The model under review builds one solid part; all positions refer to its coordinate system, in mm. A direction names the side the tool comes from. Coordinates: 2 decimals unless noted, no trailing zeros. Loops run counter-clockwise (first coordinate to the right, second up) from the corner with the lowest first, then second, coordinate; pieces in that order, holes last. Notation, with made-up numbers: M 63,1.5 L 67,1.5 A13 ccw 67,16.5 Z; hole C 77,69.5 d11. An arc over 180 degrees is marked long. Use one line per item in the form item = value.
```python
from build123d import *

# Parameters (mm, degrees)
BOSS_EXTRUDE5_DEPTH = 3
BOSS_EXTRUDE6_START = -6
BOSS_EXTRUDE6_DEPTH = 6
CIRPATTERN4_COUNT   = 12
BOSS_EXTRUDE8_START = -9
BOSS_EXTRUDE8_DEPTH = 9
SKETCH25_R          = 27.5
SKETCH25_W          = 9
SKETCH25_H          = 25
BOSS_EXTRUDE9_DEPTH = 3
CIRPATTERN5_COUNT   = 12
FILLET2_R           = 3


with BuildPart() as part:
    # Sketch1 → Boss-Extrude5 (new body)
    with BuildSketch(Plane.XY):
        with BuildLine():
            ThreePointArc((14.753571677, -27.264117862), (12.634850146, -34.380016896), (19.750749181, -36.498738428))
            ThreePointArc((19.750749181, -36.498738428), (41.5, 0), (19.750749181, 36.498738428))
            ThreePointArc((19.750749181, 36.498738428), (12.634850146, 34.380016896), (14.753571677, 27.264117862))
            ThreePointArc((14.753571677, 27.264117862), (31, 0), (14.753571677, -27.264117862))
        make_face()
    extrude(amount=BOSS_EXTRUDE5_DEPTH)

    # Sketch1<7> → Boss-Extrude6 (add)
    with BuildSketch(Plane.XY.offset(BOSS_EXTRUDE6_START)):
        with BuildLine():
            ThreePointArc((40, 0), (33.333983987, -22.109851007), (15.557724422, -36.850470972))
            ThreePointArc((15.557724422, -36.850470972), (17.691016162, -37.113053671), (19.750749181, -36.498738428))
            ThreePointArc((19.750749181, -36.498738428), (35.650428406, -21.243750952), (41.5, 0))
            ThreePointArc((41.5, 0), (35.650428406, 21.243750952), (19.750749181, 36.498738428))
            ThreePointArc((19.750749181, 36.498738428), (17.691016162, 37.113053671), (15.557724422, 36.850470972))
            ThreePointArc((15.557724422, 36.850470972), (33.333983987, 22.109851007), (40, 0))
        make_face()
    extrude(amount=BOSS_EXTRUDE6_DEPTH)

    # Sketch23 → M4x0.7 Tapped Hole4 (revolve, cut)
    with BuildSketch(Plane(origin=(36.25, 0, 3), x_dir=(0, -1, 0), z_dir=(1, 0, 0))):
        Polygon((0, 0), (0, 11.091420021), (1.65, 10.1), (1.65, 0.375), (2.025, 0), align=None)
    m4x0_7_tapped_hole4 = revolve(axis=Axis((36.25, 0, 9.35), (0, 0, -1)), mode=Mode.SUBTRACT)

    # CirPattern4: M4x0.7 Tapped Hole4 ×12 about axis, 7 skipped
    cirpattern4_axis = Axis((0, 0, 0), (0, 0, -1))
    add([m4x0_7_tapped_hole4.rotate(cirpattern4_axis, i * 360 / CIRPATTERN4_COUNT) for i in range(1, CIRPATTERN4_COUNT) if i not in (3, 4, 5, 6, 7, 8, 9)], mode=Mode.SUBTRACT)

    # Sketch15 → Boss-Extrude8 (add)
    with BuildSketch(Plane.XY.offset(3).offset(BOSS_EXTRUDE8_START)):
        with BuildLine():
            Line((47.5, 12.5), (47.5, -12.5))
            ThreePointArc((47.5, -12.5), (39.682119593, -17.947088957), (33.186389126, -24.918137506))
            ThreePointArc((33.186389126, -24.918137506), (41.5, 0), (33.186389126, 24.918137506))
            ThreePointArc((33.186389126, 24.918137506), (39.682119593, 17.947088957), (47.5, 12.5))
        make_face()
    extrude(amount=BOSS_EXTRUDE8_DEPTH)

    # Sketch25 → Boss-Extrude9 (add)
    # profile 1 of 2: a face of its own
    with BuildSketch(Plane(origin=(47.5, 0, 0), x_dir=(0, 0, -1), z_dir=(1, 0, 0))):
        with Locations((1.5, 0)):
            Circle(SKETCH25_R)
        with Locations((1.5, 0)):
            Rectangle(SKETCH25_W, SKETCH25_H, mode=Mode.SUBTRACT)
    # profile 2 of 2: a face of its own
    with BuildSketch(Plane(origin=(47.5, 0, 0), x_dir=(0, 0, -1), z_dir=(1, 0, 0))):
        with Locations((1.5, 0)):
            Rectangle(SKETCH25_W, SKETCH25_H)
    extrude(amount=BOSS_EXTRUDE9_DEPTH)

    # Sketch28 → M4x0.7 Tapped Hole5 (revolve, cut)
    with BuildSketch(Plane(origin=(50.5, 5.823428515, -23.233331092), x_dir=(0, 0, -1), z_dir=(0, 1, 0))):
        Polygon((0, 0), (0, 11.091420021), (1.65, 10.1), (1.65, 0.375), (2.025, 0), align=None)
    m4x0_7_tapped_hole5 = revolve(axis=Axis((56.85, 5.823428515, -23.233331092), (-1, 0, 0)), mode=Mode.SUBTRACT)

    # CirPattern5: M4x0.7 Tapped Hole5 ×12 about axis, 6 skipped
    cirpattern5_axis = Axis((0, -0.031748609, -1.381512577), (1, 0, 0))
    add([m4x0_7_tapped_hole5.rotate(cirpattern5_axis, i * 360 / CIRPATTERN5_COUNT) for i in range(1, CIRPATTERN5_COUNT) if i not in (2, 3, 6, 7, 10, 11)], mode=Mode.SUBTRACT)

    # Fillet2
    fillet2_edges = [part.edges().sort_by_distance(p)[0] for p in [
        (47.5, 0, -6),
        (47.5, 12.5, -1.5),
        (47.5, -12.5, -1.5),
        (47.5, 0, 3),
    ]]
    fillet(fillet2_edges, radius=FILLET2_R)


solid = part.part
```
1. Add section B-B (z = -1.5). State the section outline as (x, y) points, then the cut area to 3 significant figures.
Response values:
outline = M 15.56,-36.85 A5.25 ccw 19.75,-36.5 A41.5 ccw 33.19,-24.92 A45 cw 42.74,-15.52 A3 cw 47.5,-17.95 L 47.5,-27.5 L 50.5,-27.5 L 50.5,27.5 L 47.5,27.5 L 47.5,17.95 A3 cw 42.74,15.52 A45 cw 33.19,24.92 A41.5 ccw 19.75,36.5 A5.25 ccw 15.56,36.85 A40 cw Z
area = 546 mm^2
2. Add section C-C (y = 28.5). State the section outline as (x, z) points, then the cut area to 3 significant figures.
Response values:
outline = M 13.24,0 L 28.07,0 L 28.07,-6 L 30.17,-6 L 30.17,3 L 13.24,3 Z
area = 63.4 mm^2
3. Machinability: for faces 1 (the face through (32, 0, 0)), 2 (the face through (46.64, -0.25, 3.9)), which of the approach directions +Z, -Z, +X, -X, +Y, -Y give a long, thin tool a straight path to every point of the face, cutting with its end or side? Answer none if there is none.
Response values:
face_1 = -Z, -X
face_2 = +Z, -X, +Y, -Y
4. Insertion check: P1, Ø8.5, axis at x = 37, y = 2, coming from the -Z side; P2, Ø5.5, axis at x = 18.13, y = 31.39, coming from the -Z side; P3, Ø16.5, axis at y = -1.5, z = -2, coming from the -X side. Each pin has a flat end and moves straight along its axis. Give the tip position at first contact, or say it passes through.
Response values:
P1 = -6
P2 = 0
P3 = 29.51
5. Add section D-D (x = 36.25). State the section outline as (y, z) points (3 decimals).
Response values:
outline = M -21.259,-6 L -16.91,-6 L -16.91,0 L -1.65,0 L -1.65,2.625 L -2.025,3 L -21.259,3 Z; M 1.65,0 L 16.91,0 L 16.91,-6 L 21.259,-6 L 21.259,3 L 2.025,3 L 1.65,2.625 Z
6. The part is to be moulded in two halves that separate along Y. For faces 3 (the face through (46.5, 15.71, -1.39)), 4 (the face through (31.036, -16.514, 1.331)), 5 (the face through (46.64, -0.25, -6.9)), say which applies: pulls with the +Y half, pulls with the -Y half, needs draft (parallel to the pull), parting line crosses it, or undercut.
Response values:
face_3 = pulls with the +Y half
face_4 = undercut
face_5 = needs draft
7. Add section A-A (x = 23). State the section outline as (y, z) points, then the cut area to 3 significant figures.
Response values:
outline = M -34.54,-6 L -32.73,-6 L -32.73,0 L -20.78,0 L -20.78,3 L -34.54,3 Z; M 20.78,0 L 32.73,0 L 32.73,-6 L 34.54,-6 L 34.54,3 L 20.78,3 Z
area = 104 mm^2
8. Wall thickness on line 1 along Z through (x, y) = (42, -0.5); line 2 along Z through (x, y) = (31, -3.5); line 3 along X through (y, z) = (13, 13.5): over which ranges is each line inside the solid? List them lowest first. Write a range as from..to.
Response values:
line_1 = -6..3
line_2 = 0..3
line_3 = 47.5..50.5
